Can you work these out from the model? Positions are in its coordinate system, mm. Face numbers are marked on the shaded views. A direction names the side the tool comes from. Round coordinates to 2 decimals unless told otherwise and drop trailing zeros. Loops run counter-clockwise (first coordinate to the right, second up) from the corner with the lowest first, then second, coordinate; pieces in that order, holes last. Notation, with made-up numbers: M -34,79.25 L -18,79.25 A34 ccw -18,111.25 Z; hole C 41,25.25 d10. An arc over 180 degrees is marked long. Answer as CSV lines item,"result".
from build123d import *

# Parameters (mm, degrees)
BOSS_EXTRUDE1_DEPTH     = 33.02
BOSS_EXTRUDE2_DEPTH     = 76.2
CUT_EXTRUDE1_REACH      = 150.106
CUT_EXTRUDE2_DEPTH      = 149.106178129
CUT_EXTRUDE2_DEPTH_BACK = 149.106178129


with BuildPart() as part:
    # Sketch1 → Boss-Extrude1 (new body)
    with BuildSketch(Plane.XY):
        Polygon((-76.2, 50.8), (-76.2, 0), (0, 76.2), (0, 101.6), (-25.4, 101.6), align=None)
        Polygon((0, 101.6), (0, 76.2), (76.2, 0), (76.2, 50.8), (25.4, 101.6), align=None)
        Polygon((0, 76.2), (0, 0), (76.2, 0), align=None)
        Polygon((0, 76.2), (-76.2, 0), (0, 0), align=None)
    extrude(amount=-BOSS_EXTRUDE1_DEPTH)

    # Sketch2 → Boss-Extrude2 (add)
    with BuildSketch(Plane(origin=(0, 0, 0), x_dir=(1, 0, 0), z_dir=(0, 1, 0))):
        Polygon((-76.2, 0), (-76.2, -76.2), (-38.1, -76.2), (-38.1, -50.8), (38.1, -50.8), (38.1, -76.2), (76.2, -76.2), (76.2, 0), align=None)
    extrude(amount=BOSS_EXTRUDE2_DEPTH)

    # Sketch1<5> → Cut-Extrude1 (cut, up to next)
    with BuildSketch(Plane.XY, mode=Mode.PRIVATE) as cut_extrude1_sk1:
        Polygon((-76.2, 50.8), (-76.2, 0), (0, 76.2), (0, 101.6), (-25.4, 101.6), align=None)
    cut_extrude1_tool1 = extrude(cut_extrude1_sk1.sketch, amount=CUT_EXTRUDE1_REACH, mode=Mode.PRIVATE) & part.part
    # Sketch1<5> → Cut-Extrude1 (cut, up to next)
    with BuildSketch(Plane.XY, mode=Mode.PRIVATE) as cut_extrude1_sk2:
        Polygon((0, 101.6), (0, 76.2), (76.2, 0), (76.2, 50.8), (25.4, 101.6), align=None)
    cut_extrude1_tool2 = extrude(cut_extrude1_sk2.sketch, amount=CUT_EXTRUDE1_REACH, mode=Mode.PRIVATE) & part.part
    add(cut_extrude1_tool1.solids().sort_by_distance((-40.793939, 59.266667, 0))[0], mode=Mode.SUBTRACT)
    add(cut_extrude1_tool2.solids().sort_by_distance((40.793939, 59.266667, 0))[0], mode=Mode.SUBTRACT)


with BuildPart() as body_2:
    # of the pieces the cut leaves, the one that is kept (cut_extrude1_keep)
    add(part.part.solids().sort_by_distance((-25.4, 101.6, 0))[0])

    # Sketch6 → Cut-Extrude2 (cut, two sides)
    with BuildSketch(Plane(origin=(0, 0, 0), x_dir=(0, 0, -1), z_dir=(1, 0, 0))) as cut_extrude2_sk:
        Polygon((-76.2, 0), (0, 76.2), (-76.2, 76.2), align=None)
    extrude(amount=CUT_EXTRUDE2_DEPTH, mode=Mode.SUBTRACT)
    extrude(cut_extrude2_sk.sketch, amount=-CUT_EXTRUDE2_DEPTH_BACK, mode=Mode.SUBTRACT)


solid = body_2.part
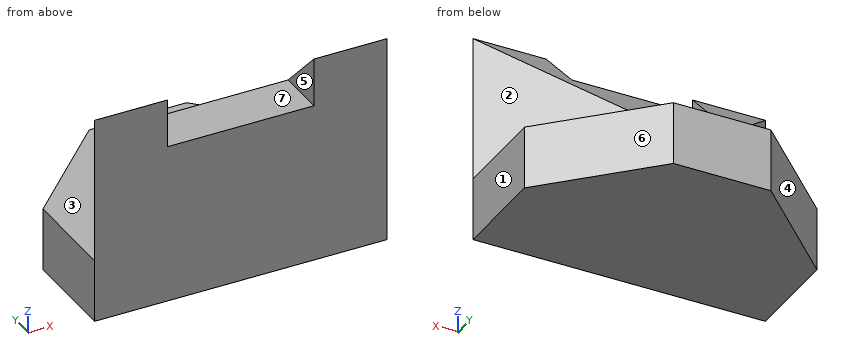
Item 1: If we section it at B-B on x = -65: Write out the boundary of the cut face in (y, z).
Output:
outline,"M 0,-33.02 L 62,-33.02 L 62,0 L 11.2,0 L 11.2,65 L 0,76.2 Z"
Item 2: If we section it at A-A on y = 60.5: Write out the boundary of the cut face in (x, z), then the cut area to 3 significant figures.
Output:
outline,"M -66.5,-33.02 L 66.5,-33.02 L 66.5,0 L 15.7,0 L 15.7,15.7 L -15.7,15.7 L -15.7,0 L -66.5,0 Z"
area,"4,880 mm2"
Item 3: Will these pins go through, and if not, where does the flat tip stop? pin 1 (1 mm diameter, centred on y = 20.5, z = 51.5, fed in from +X); pin 2 (1.5 mm diameter, centred on x = -16, y = 75.5, fed in from +Z); pin 3 (10 mm diameter, centred on x = -58.5, z = 46, fed in from +Y).
Output:
pin 1,"stops at x = 56.2"
pin 2,"stops at z = 0"
pin 3,"stops at y = 22.7"
Item 4: On a 3-axis mill with a long thin cutter (end or side, diameter ignored), from which of +Z, -Z, +X, -X, +Y, -Y can I reach the whole of each face in a straight line? I mean the marked faces 1, 2 and 3. Say none if no direction works.
Output:
face 1,"+Z, -Z, +X, +Y, -Y"
face 2,"+Z, +X, +Y"
face 3,"+Z, +Y"
Item 5: If I drill on line 1 along Z through (x, y) = (16.5, 88); line 2 along Z through (x, y) = (-23, 19); line 3 along Y through (x, z) = (-54.5, -13), over which ranges is the centre line in solid material (lowest first)? Write a range as from..to.
Output:
line 1,"z = -33.02..0"
line 2,"z = -33.02..50.8"
line 3,"y = 0..72.5"
Item 6: We'd pull the mould along X, two halves only. Please class the marked faces 4, 5, 6 and 7: released by +X, released by -X, zero draft, split by the parting line, or undercut.
Output:
face 4,"released by -X"
face 5,"undercut"
face 6,"released by +X"
face 7,"undercut"
Item 7: If we section it at C-C on z = -16.5: Write out the boundary of the cut face in (x, y).
Output:
outline,"M -76.2,0 L 76.2,0 L 76.2,50.8 L 25.4,101.6 L -25.4,101.6 L -76.2,50.8 Z"
Item 8: If we section it at D-D on y = 31: Write out the boundary of the cut face in (x, z), then the cut area to 3 significant figures.
Output:
outline,"M -76.2,-33.02 L 76.2,-33.02 L 76.2,0 L 45.2,0 L 45.2,45.2 L -45.2,45.2 L -45.2,0 L -76.2,0 Z"
area,"9,120 mm2"
